Autodesk Inventor part; units mm, degrees
ref_plane "YZ Plane" through (0, 0, 0) normal (1, 0, 0) x (0, 1, 0)
ref_plane "XZ Plane" through (0, 0, 0) normal (0, 1, 0) x (-1, 0, 0)
ref_plane "XY Plane" through (0, 0, 0) normal (0, 0, 1) x (1, 0, 0)
sketch "Sketch1" plane through (0, 0, 0) normal (0, 0, 1) x (1, 0, 0)
  circle A0 centre (0, 0) radius 3.35
  circle A1 centre (0, 0) radius 2
  dimension "d0" = 6.7
  dimension "d1" = 4
extrude "Extrusion1" add sketch "Sketch1" along normal blind 5
sketch "Sketch2" plane through (0, 0, 5) normal (0, 0, 1) x (1, 0, 0)
  circle A0 centre (0, 0) radius 2
  circle A1 centre (0, 0) radius 3.35
  circle A2 centre (0, 0) radius 4.5
  dimension "d4" = 6.7
  dimension "d5" = 9
extrude "Extrusion2" add sketch "Sketch2" along normal blind 5 and the other way blind 2 contours A2
chamfer "Chamfer1" distance 1 angle 45 2 edges at (-4.5, 0, 3) (-2, 0, 5)
properties part number "Matchboxscope_lenstube_v0"
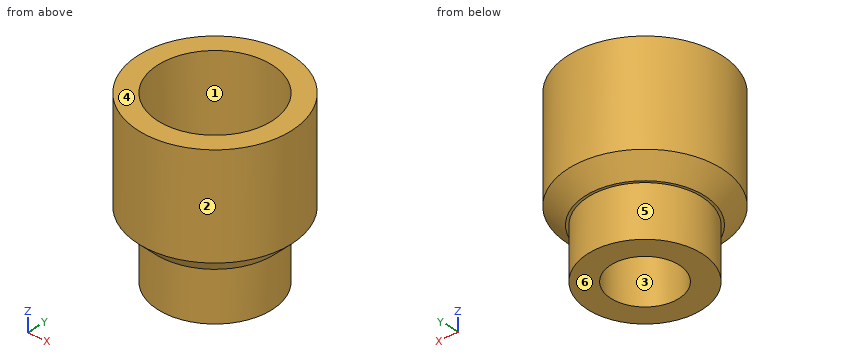
Model file for the job. Use its own axes, mm. Face numbers are marked on the shaded views. A direction names the side the tool comes from. Coordinates: 2 decimals unless noted, no trailing zeros. Loops run counter-clockwise (first coordinate to the right, second up) from the corner with the lowest first, then second, coordinate; pieces in that order, holes last. Notation, with made-up numbers: (21, -19.5) - (58, -19.5) arc R13 cw to (58, -3.5) - close; hole circle Ø6 at (17, 0). An arc over 180 degrees is marked (long way). Answer as a JSON object with one key per item and string values. Group by question number.
(1) Cut at A-A (x = 0). Give the cut face in (y, z), then the cut area to 3 significant figures.
(2) Cut at C-C (z = 3.25). Give the cut face in (x, y), then the cut area to 3 significant figures.
(3) Tool access for the marked faces 5 and 6: list every direction of +Z, -Z, +X, -X, +Y, -Y with a clear straight run to the whole face (end or side of a thin tool).
(4) Two-plate mould, pull along X, no slides. Class the marked faces 1, 2, 3 and 4: released by +X, released by -X, zero draft, split by the parting line, or undercut.
(5) Cut at D-D (z = 9). Give the cut face in (x, y).
(6) Flat gauge pins, fed straight in: pin 1 (4 mm diameter, centred on y = 3, z = 3, fed in from -X); pin 2 (1 mm diameter, centred on x = 3.5, z = 5.5, fed in from -Y); pin 3 (2 mm diameter, centred on y = 3, z = 4.5, fed in from -X); pin 4 (2.5 mm diameter, centred on x = 0, y = 0, fed in from +Z). Where does each tip first touch, or does it go through?
(7) Probe line 1 along Y through (x, z) = (0, 2.85); line 2 along Y through (x, z) = (0, 8.45); line 3 along X through (y, z) = (2.25, 7.5). List the from-to ranges inside material, lowest first.
Geometry says:
{
 "1": {"outline": "(-4.5, 4) - (-3.5, 3) - (-3.35, 3) - (-3.35, 0) - (-2, 0) - (-2, 4) - (-3, 5) - (-3.35, 5) - (-3.35, 10) - (-4.5, 10) - close; (2, 0) - (3.35, 0) - (3.35, 3) - (3.5, 3) - (4.5, 4) - (4.5, 10) - (3.35, 10) - (3.35, 5) - (3, 5) - (2, 4) - close", "area": "27.6 mm^2"},
 "2": {"outline": "circle Ø7.5 at (0, 0); hole circle Ø4 at (0, 0)", "area": "31.6 mm^2"},
 "3": {"face 5": "-Z", "face 6": "-Z, +X, -X, +Y, -Y"},
 "4": {"face 1": "undercut", "face 2": "split by the parting line", "face 3": "undercut", "face 4": "zero draft"},
 "5": {"outline": "circle Ø9 at (0, 0); hole circle Ø6.7 at (0, 0)"},
 "6": {"pin 1": "stops at x = -4.32", "pin 2": "stops at y = -3.35", "pin 3": "stops at x = -4.03", "pin 4": "passes through"},
 "7": {"line 1": "y = -3.35 to -2, 2 to 3.35", "line 2": "y = -4.5 to -3.35, 3.35 to 4.5", "line 3": "x = -3.9 to -2.48, 2.48 to 3.9"}
}
